Autodesk Inventor part; units mm, degrees
ref_plane "Work Plane1" through (29, 0, 0) normal (0, -1, 0) x (1, 0, 0)
ref_plane "YZ Plane" through (0, 0, 0) normal (1, 0, 0) x (0, 1, 0)
ref_plane "XZ Plane" through (0, 0, 0) normal (0, 1, 0) x (-1, 0, 0)
sketch "Эскиз1" plane through (0, 0, 0) normal (0, 0, 1) x (1, 0, 0)
  line L0 (-1, 0) -> (6, 0)
  line L1 (6, 0) -> (6, 2)
  line L2 (6, 2) -> (2.1, 2)
  line L3 (2.1, 2) -> (1.6705, 1.7853)
  line L4 (1.6705, 1.7853) -> (0, 1.7853)
  line L5 (0, 1.7853) -> (0, 3.5)
  line L6 (0, 3.5) -> (-4, 3.5)
  line L7 (-4, 3.5) -> (-4, 1.7321)
  line L8 (-4, 1.7321) -> (-2, 1.7321)
  line L9 (-2, 1.7321) -> (-1, 0)
  line L10 (-6, 0) -> (8, 0)
  line L11 (0, -0.7) -> (0, 4.2)
  line L12 (2.1, 2) -> (0, 2) construction
  dimension "d1" = 3.9
  dimension "d2" = 0.4295
  dimension "d3" = 4
  dimension "d4" = 2
  dimension "d5" = 60
  dimension "d6" = 4
  dimension "d7" = 3.5705
  dimension "d8" = 3.4641
  dimension "d9" = 7
  dimension "d26" = 6
revolve "Базовый элемент" add sketch "Эскиз1" angle 360 about axis through (-1, 0, 0) along (1, 0, 0)
sketch "Эскиз2" plane through (-4, 0, 0) normal (-1, 0, 0) x (0, 0, 1)
  circle A0 centre (0, 0) radius 1.7321
  line L0 (0, -4.9) -> (0, 4.9)
  line L1 (-4.9, 0) -> (4.9, 0)
  line L2 (1.7321, 0) -> (0.866, -1.5)
  line L3 (0.866, -1.5) -> (-0.866, -1.5)
  line L4 (-0.866, -1.5) -> (-1.7321, 0)
  line L5 (-1.7321, 0) -> (-0.866, 1.5)
  line L6 (-0.866, 1.5) -> (0.866, 1.5)
  line L7 (0.866, 1.5) -> (1.7321, 0)
extrude "Паз" add sketch "Эскиз2" against normal up to next contours L7 A0 | A0 L2 | L6 L0 A0 | A0 L0 L3 | L0 L6 A0 | A0 L3 L0 | L4 A0 | A0 L5
fillet "Сопряжение1" radius 0.4 1 edges at (-4, -3.5, 0)
thread "Резьба"
chamfer "Фаска1" distance 0.4294 distance2 0.4294 1 edges at (6, -2, 0) measured on face at (6, 0.556, 0.0273)
ref_plane "Work Plane1" through (29, 0, 0) normal (0, -1, 0) x (1, 0, 0)
fillet "Fillet2" radius 0.1 1 edges at (0, -1.7853, 0)
equation "\"d1\" = GEL"
equation "\"d3\" = KOH"
equation "\"d4\" = INTI"
equation "\"d6\" = GD"
equation "\"d7\" = BDM"
equation "\"d8\" = 1.1547 * SW"
equation "\"d9\" = KOD"
equation "\"d26\" = NLG"
equation "\"d30\" = R"
equation "\"d17\" = RR"
equation "\"d13\" = GEL"
equation "\"d15\" = -0.5 * SPD + 0.5 * GD"
equation "\"d16\" = GUL"
equation "\"GD\" = NND"
equation "\"NLG\" = 6"
equation "\"GEL\" = 3.9"
equation "\"KOD\" = 7"
equation "\"KOH\" = NND"
equation "\"INTI\" = 2"
equation "\"GAL\" = 0.61345 * PTC"
equation "\"GUL\" = 0.61345 * PTC"
equation "\"BDM\" = 3.5705"
equation "\"SW\" = 3"
equation "\"RR\" = 0.4"
equation "\"SPD\" = NND - 1.2269 * PTC"
equation "\"R\" = 0.1"
equation "\"PHH\" = 0.4"
equation "\"GD1\" = THREADDIA - 1.2269 * PTC"
equation "\"THREADDIA\" = 4"
equation "\"FAWI\" = 45deg"
equation "\"PTC\" = 0.7"
equation "\"NND\" = 4"
equation "\"TOA\" = 30deg"
equation "\"E0\" = 1.155 * SW"
properties part number "CSN 02 1143 - M4 x 6" material "Сталь, мягкая"
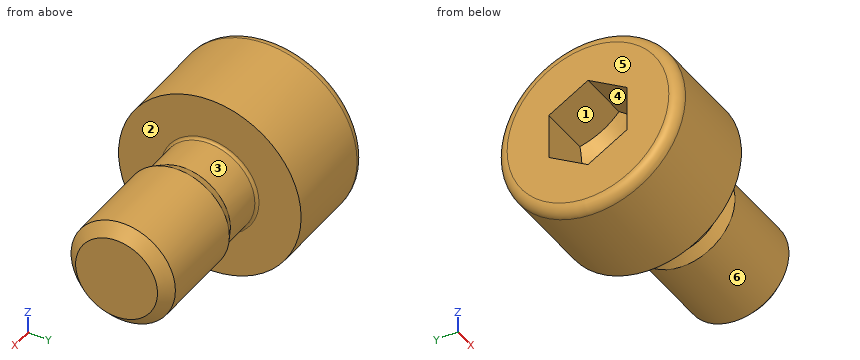
Source: CAD feature listing. Evaluate the final solid. Frame: model axes, mm. Face numbers are marked on the shaded views. A direction names the side the tool comes from. Give positions to 0.01 mm unless a question says otherwise; leave off trailing zeros. Write each loop counter-clockwise with the first axis right and the second up, starting at its lowest first coordinate (ties: lowest second). Pieces come first, ordered by that corner, then holes. Notation, with made-up numbers: M -27,-15.75 L -11,-15.75 A29 cw -11,7.25 Z; hole C -34.5,50.25 d3. An arc over 180 degrees is marked long. Return JSON: item names as keys, results as strings. Group by question number.
1) Set-up query: the marked faces 4, 5 and 6. Return all of +Z, -Z, +X, -X, +Y, -Y with unobstructed straight access to the full face (end or side cutting, diameter ignored); none if empty.
2) Pull-direction query (Y, two-part tool) for the marked faces 1, 2 and 3; classes: pulls with the +Y half, pulls with the -Y half, needs draft (parallel to the pull), parting line crosses it, or undercut.
3) Cut plane A-A, the plane x = -2.25. Output: boundary loops of the cut face in (y, z), plus the area to 3 significant figures.
4) Material intervals for line 1 along X through (y, z) = (1.75, -2.5); line 2 along Z through (x, y) = (-3.5, -1.25); line 3 along Z through (x, y) = (-1.5, -0.25), sorted ascending. Write a range as [from, to].
5) Cut plane B-B, the plane x = 0.25. Output: boundary loops of the cut face in (y, z), plus the area to 3 significant figures.
Recorded:
{
 "1": {"face 4": "-X", "face 5": "+Z, -Z, -X, +Y, -Y", "face 6": "+X"},
 "2": {"face 1": "undercut", "face 2": "needs draft", "face 3": "parting line crosses it"},
 "3": {"outline": "C 0,0 d7; hole M -1.5,-0.87 L 0,-1.73 L 1.5,-0.87 L 1.5,0.87 L 0,1.73 L -1.5,0.87 Z", "area": "30.7 mm²"},
 "4": {"line 1": "x = [-4, 0]", "line 2": "z = [-3.27, -1.01], [1.01, 3.27]", "line 3": "z = [-3.49, -0.83], [0.83, 3.49]"},
 "5": {"outline": "C 0,0 d3.57", "area": "10.0 mm²"}
}
